Part model, mm, in its own coordinate system. Face numbers are marked on the shaded views. A direction names the side the tool comes from. Round coordinates to 2 decimals unless told otherwise and drop trailing zeros. Write each loop counter-clockwise with the first axis right and the second up, starting at its lowest first coordinate (ties: lowest second). Pieces come first, ordered by that corner, then holes. Notation, with made-up numbers: M -36,-38.75 L 0,-38.75 A22 cw 0,-24.75 Z; hole C -9.5,18 d8. An arc over 180 degrees is marked long. Use one line per item in the form item = value. Start each with the question number.
Item 1: Flat gauge pins, fed straight in: pin 1 Ø10 at (y, z) = (16.5, 31) entering from +X; pin 2 Ø3.5 at (x, y) = (49.5, 18) entering from +Z; pin 3 Ø12 at (x, y) = (39.5, 14) entering from +Z. Where does each tip first touch, or does it go through?
Item 2: Cut at A-A, the plane x = 50.8. Give the cut face in (y, z).
Item 3: Probe L1, parallel to Z at x = 51.5, y = 1.5; L2, parallel to Z at x = 54, y = 15; L3, parallel to X at y = 3.5, z = 4.5. List the from-to ranges inside material, lowest first.
Item 4: Which spindle directions (+Z, -Z, +X, -X, +Y, -Y) get a long thin tool onto all of the face, cutting with end or side? Do the marked faces 1 and 2. Say none if no direction does.
Item 5: Cut at B-B, the plane y = 13.75. Give the cut face in (x, z).
Item 6: Mould opens along Y. For the marked faces 3, 4 and 5 say: +Y half, -Y half, draft (parallel to the pull), parting line (faces both ways), or undercut.
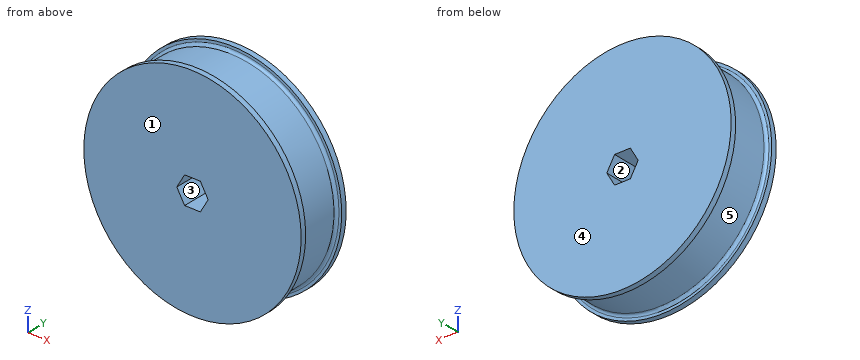
Autodesk Inventor part; units mm, degrees
ref_plane "YZ Plane" through (0, 0, 0) normal (1, 0, 0) x (0, 1, 0)
ref_plane "XZ Plane" through (0, 0, 0) normal (0, 1, 0) x (-1, 0, 0)
ref_plane "XY Plane" through (0, 0, 0) normal (0, 0, 1) x (1, 0, 0)
sketch "Sketch1" plane through (0, 0, 0) normal (0, 0, 1) x (1, 0, 0)
  line L0 (0, 0) -> (50.8, 0)
  line L1 (50.8, 0) -> (50.8, 25.4)
  line L2 (50.8, 25.4) -> (0, 25.4)
  line L3 (0, 25.4) -> (0, 0)
  line L4 (0, 22.86) -> (1.27, 22.86)
  line L5 (2.54, 21.59) -> (2.54, 3.81)
  line L6 (1.27, 2.54) -> (0, 2.54)
  arc A0 (2.54, 21.59) -> (1.27, 22.86) centre (1.27, 21.59) ccw
  arc A1 (1.27, 2.54) -> (2.54, 3.81) centre (1.27, 3.81) ccw
  point P0 (0.635, 22.86)
  point P1 (0.635, 2.54)
  point P2 (41.91, 0)
  point P3 (41.91, 25.4)
  dimension "d0" = 50.8
  dimension "d1" = 25.4
  dimension "d2" = 2.54
  dimension "d3" = 2.54
  dimension "d4" = 2.54
  dimension "d5" = 1.27
revolve "Revolution1" add sketch "Sketch1" angle 360 about axis through (50.8, 0, 0) along (0, 1, 0) contours L3 L6 A1 L5 A0 L4 L2 L1 L0
sketch "Sketch2" plane through (50.8, 25.4, 0) normal (0, 1, 0) x (1, 0, 0)
  circle A0 centre (0, 0) radius 50.8
  point P0 (-50.8, 0)
sketch "Sketch3" plane through (50.8, 25.4, 0) normal (0, 1, 0) x (1, 0, 0)
  circle A0 centre (0, 0) radius 6.35
  circle A1 centre (0, 0) radius 50.8
  line L0 (3.6662, 6.35) -> (7.3323, 0)
  line L1 (7.3323, 0) -> (3.6662, -6.35)
  line L2 (3.6662, -6.35) -> (-3.6662, -6.35)
  line L3 (-3.6662, -6.35) -> (-7.3323, 0)
  line L4 (-7.3323, 0) -> (-3.6662, 6.35)
  line L5 (-3.6662, 6.35) -> (3.6662, 6.35)
  point P0 (-50.8, 0)
  point P1 (0, 6.35)
  dimension "d9" = 12.7
extrude "Extrusion1" cut sketch "Sketch3" against normal blind 25.4 contours A0 | A0 L0 L1 | A0 L5 L0 | L1 L2 A0 | A0 L4 L5 | L2 L3 A0 | A0 L3 L4
properties part number "4-bar intake () pully"
Model answer:
q1.pin_1 = 91.46
q1.pin_2 = 48.26
q1.pin_3 = 47.97
q2.outline = M 0,-50.8 L 2.54,-50.8 L 2.54,-49.53 A1.27 cw 3.81,-48.26 L 21.59,-48.26 A1.27 cw 22.86,-49.53 L 22.86,-50.8 L 25.4,-50.8 L 25.4,-6.35 L 0,-6.35 Z; M 0,6.35 L 25.4,6.35 L 25.4,50.8 L 22.86,50.8 L 22.86,49.53 A1.27 cw 21.59,48.26 L 3.81,48.26 A1.27 cw 2.54,49.53 L 2.54,50.8 L 0,50.8 Z
q3.L1 = -50.8 to -6.35, 6.35 to 50.8
q3.L2 = -48.15 to -6.35, 6.35 to 48.15
q3.L3 = 2.71 to 46.07, 55.53 to 98.89
q4.face_1 = +Z, -Z, +X, -X, -Y
q4.face_2 = +Y, -Y
q5.outline = C 50.8,0 d96.52; hole M 43.47,0 L 47.13,-6.35 L 54.47,-6.35 L 58.13,0 L 54.47,6.35 L 47.13,6.35 Z
q6.face_3 = draft
q6.face_4 = +Y half
q6.face_5 = undercut
